```python
from build123d import *

# Parameters (mm, degrees)
F0_W     = 533.4
F0_H     = 101.6
F1_DEPTH = 25.4
F2_W     = 127
F2_H     = 50.8
F3_DEPTH = 50.8
F4_R     = 5.08


with BuildPart() as f1:
    # F0 (on Front) → F1 (new body)
    with BuildSketch(Plane.XZ):
        with Locations((-266.7, -50.8)):
            Rectangle(F0_W, F0_H)
    extrude(amount=F1_DEPTH)

    # F2 (on face) → F3 (cut)
    with BuildSketch(Plane.XZ.offset(25.4)):
        with Locations((-241.3, -50.8)):
            Rectangle(F2_W, F2_H)
    extrude(amount=-F3_DEPTH, mode=Mode.SUBTRACT)

    # F4
    f4_edges = [f1.edges().sort_by_distance(p)[0] for p in [
        (0, -25.4, -50.8),
        (-266.7, -25.4, -101.6),
        (-266.7, -25.4, 0),
        (-533.4, -25.4, -50.8),
        (-304.8, -25.4, -50.8),
        (-241.3, -25.4, -76.2),
        (-177.8, -25.4, -50.8),
        (-241.3, -25.4, -25.4),
    ]]
    fillet(f4_edges, radius=F4_R)


solid = f1.part
```
Input: part model. Units: mm. Frame: model coordinates. A direction names the side the tool comes from. Give positions to 0.01 mm unless a question says otherwise; leave off trailing zeros. Order: outer loops, then holes, each group sorted by start corner. A loop starts at its lowest first (then second) coordinate and runs counter-clockwise, first axis right, second up.
1. Mould query, pull axis X, two halves, no side actions, for faces 1 (the flat face through (-270, -25.4, -20)), 2 (the flat face through (-304.8, -10, -51)), 3 (the flat face through (-533.4, -10, -52)). Classes: released by +X, released by -X, zero draft, split by the parting line, or undercut.
Derived:
face 1: zero draft
face 2: undercut
face 3: released by -X
2. Material intervals for L1, parallel to Z at x = -240.5, y = -4.25; L2, parallel to X at y = -5.5, z = -52; L3, parallel to Z at x = -336.5, y = -21.25, sorted ascending.
Derived:
L1: z = -101.6 to -76.2, -25.4 to 0
L2: x = -533.4 to -304.8, -177.8 to 0
L3: z = -101.51 to -0.09
3. Section A-A on z = -41. Return the cut outline in (x, y).
Derived:
outline: (-533.4, -20.32) arc R5.08 ccw to (-528.32, -25.4) - (-309.88, -25.4) arc R5.08 ccw to (-304.8, -20.32) - (-304.8, 0) - (-533.4, 0) - close; (-177.8, -20.32) arc R5.08 ccw to (-172.72, -25.4) - (-5.08, -25.4) arc R5.08 ccw to (0, -20.32) - (0, 0) - (-177.8, 0) - close
4. Section B-B on x = -269.5. Return the cut outline in (y, z), and give its area (3 significant figures).
Derived:
outline: (-25.4, -96.52) arc R5.08 ccw to (-20.32, -101.6) - (0, -101.6) - (0, -76.2) - (-20.32, -76.2) arc R5.08 ccw to (-25.4, -81.28) - close; (-25.4, -20.32) arc R5.08 ccw to (-20.32, -25.4) - (0, -25.4) - (0, 0) - (-20.32, 0) arc R5.08 ccw to (-25.4, -5.08) - close
area: 1,270 mm2
5. Section C-C on y = -9.75. Return the cut outline in (x, z).
Derived:
outline: (-533.4, -101.6) - (0, -101.6) - (0, 0) - (-533.4, 0) - close; hole (-304.8, -76.2) - (-177.8, -76.2) - (-177.8, -25.4) - (-304.8, -25.4) - close
6. Reachability of faces 4 (the flat face through (0, -10, -52)), 5 (the flat face through (-242, -10, -25.4)) from +Z, -Z, +X, -X, +Y, -Y: full face, straight path, thin tool, end or side. Return the list, or none.
Derived:
face 4: +Z, -Z, +X, +Y, -Y
face 5: +Y, -Y
